The model under review builds one solid part; all positions refer to its coordinate system, in mm. Face numbers are marked on the shaded views. A direction names the side the tool comes from. Give positions to 0.01 mm unless a question says otherwise; leave off trailing zeros. Order: outer loops, then holes, each group sorted by start corner. A loop starts at its lowest first (then second) coordinate and runs counter-clockwise, first axis right, second up.
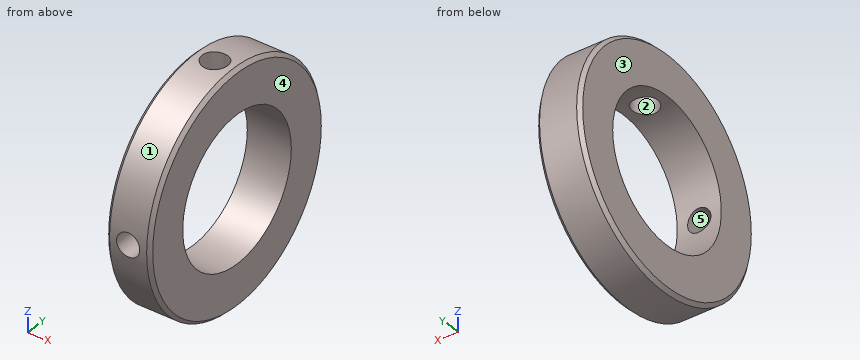
```python
from build123d import *

# Parameters (mm, degrees)
F0_R     = 25.4
F0_R_2   = 15.875
F1_DEPTH = 9.652
F2_SIZE  = 0.762
F7_SIZE  = 0.762
F8_D     = 5.55752
F8_DEPTH = 16.51
F8_TIP   = 1.6696474537
F9_D     = 5.1054
F9_DEPTH = 16.51
F9_TIP   = 1.5338169022


with BuildPart() as f1:
    # F0 (on Right) → F1 (new body)
    with BuildSketch(Plane.YZ):
        Circle(F0_R)
        Circle(F0_R_2, mode=Mode.SUBTRACT)
    extrude(amount=F1_DEPTH)

    # F2
    f2_edges = [f1.edges().sort_by_distance(p)[0] for p in [
        (9.652, -25.4, 0),
    ]]
    chamfer(f2_edges, length=F2_SIZE)

    # F7
    f7_edges = [f1.edges().sort_by_distance(p)[0] for p in [
        (0, -25.4, 0),
    ]]
    chamfer(f7_edges, length=F7_SIZE)

    # F8
    with Locations(Plane.XY.offset(25.4)):
        with Locations((4.826, 0)):
            Hole(F8_D / 2, depth=F8_DEPTH)
            with Locations((0, 0, -(F8_DEPTH + F8_TIP / 2))):  # 118° drill point
                Cone(0, F8_D / 2, F8_TIP, mode=Mode.SUBTRACT)

    # F9
    with Locations(Plane.XZ.offset(25.4)):
        with Locations((4.826, 0)):
            Hole(F9_D / 2, depth=F9_DEPTH)
            with Locations((0, 0, -(F9_DEPTH + F9_TIP / 2))):  # 118° drill point
                Cone(0, F9_D / 2, F9_TIP, mode=Mode.SUBTRACT)


solid = f1.part
```
Item 1: For line 1 (Y direction, x = 7.5, z = 0) (3 decimals); line 2 (Z direction, x = 1.5, y = -14); line 3 (Z direction, x = 7.25, y = -11), list the stretches that pass through material, from the lowest coordinate up.
Values found:
line 1: y = -25.4 to -15.875, 15.875 to 25.4
line 2: z = -21.19 to -7.48, 7.48 to 21.19
line 3: z = -22.89 to -11.45, 11.45 to 22.89
Item 2: Draft analysis for pull direction Y (two halves, no side actions). For the marked faces 1, 2 and 3, state which applies: released by +Y, released by -Y, zero draft, split by the parting line, or undercut.
Values found:
face 1: split by the parting line
face 2: undercut
face 3: zero draft
Item 3: For the marked faces 4 and 5, list the 3-axis set-ups (+Z, -Z, +X, -X, +Y, -Y) from which the entire face can be reached by the end or side of a thin tool; tool diameter is ignored.
Values found:
face 4: +Z, -Z, +X, +Y, -Y
face 5: -Y
Item 4: Take a section at A-A (y = 0). Give the boundary of the cut face in (x, z) (3 decimals), and give its area (3 significant figures).
Values found:
outline: (0, -24.638) - (0.762, -25.4) - (8.89, -25.4) - (9.652, -24.638) - (9.652, -15.875) - (0, -15.875) - close; (0, 15.875) - (2.047, 15.875) - (2.047, 25.4) - (0.762, 25.4) - (0, 24.638) - close; (7.605, 15.875) - (9.652, 15.875) - (9.652, 24.638) - (8.89, 25.4) - (7.605, 25.4) - close
area: 130 mm2
Item 5: Clearance check with flat-ended pins moving along their axes: pin 1 Ø1.5 at (x, z) = (5, 6) entering from +Y; pin 2 Ø5 at (x, z) = (2, -7) entering from +Y; pin 3 Ø2 at (y, z) = (5.5, -15.5) entering from -X; pin 4 Ø3 at (x, z) = (6.5, 8) entering from +Y. State where each tip first meets the part, or that it passes through.
Values found:
pin 1: stops at y = 24.85
pin 2: stops at y = 25
pin 3: stops at x = 0
pin 4: stops at y = 24.55
Item 6: Take a section at B-B (z = 0). Give the boundary of the cut face in (x, y) (3 decimals), and give its area (3 significant figures).
Values found:
outline: (0, -24.638) - (0.762, -25.4) - (2.273, -25.4) - (2.273, -15.875) - (0, -15.875) - close; (0, 15.875) - (9.652, 15.875) - (9.652, 24.638) - (8.89, 25.4) - (0.762, 25.4) - (0, 24.638) - close; (7.379, -25.4) - (8.89, -25.4) - (9.652, -24.638) - (9.652, -15.875) - (7.379, -15.875) - close
area: 134 mm2
Item 7: Take a section at C-C (x = 3.5). Give the boundary of the cut face in (y, z) (3 decimals).
Values found:
outline: (-25.306, -2.181) arc R25.4 ccw (long way) to (2.442, 25.282) - (2.442, 15.686) arc R15.875 cw (long way) to (-15.724, -2.181) - close; (-25.306, 2.181) - (-15.724, 2.181) arc R15.875 cw to (-2.442, 15.686) - (-2.442, 25.282) arc R25.4 ccw to start
